Here's how the part is built. I have some questions about the finished solid (model axes, mm). A direction names the side the tool comes from. Give positions to 0.01 mm unless a question says otherwise; leave off trailing zeros. Write each loop counter-clockwise with the first axis right and the second up, starting at its lowest first coordinate (ties: lowest second). Pieces come first, ordered by that corner, then holes. Notation, with made-up numbers: M 40,-37 L 71,-37 A29 cw 71,-15 Z; hole C 34,33 d3. An arc over 180 degrees is marked long. Answer as CSV lines item,"result". Start each with the question number.
Q1. Suppose I cut it at C-C (z = 22). Write out the boundary of the cut face in (x, y).
Q2. Thinking about a two-plate mould opening in Y: for faces 1 (the cylindrical face through (5.009, -4.303, -13.206)), 2 (the cylindrical face through (6.26, -11.93, -10.25)), 3 (the cylindrical face through (6.26, 11.96, -10.3)), 4 (the cylindrical face through (5.009, 1.304, 15.728)), which applies, +Y half, -Y half, draft (parallel to the pull), parting line (faces both ways), or undercut?
Q3. Suppose I cut it at B-B (y = 0). Write out the boundary of the cut face in (x, z), then the cut area to 3 significant figures.
Q4. On a 3-axis mill with a long thin cutter (end or side, diameter ignored), from which of +Z, -Z, +X, -X, +Y, -Y can I reach the whole of each face in a straight line? I mean faces 5 (the cylindrical face through (6.261, -14.555, 6.101)), 6 (the flat face through (12.7, 0, 0)), 7 (the cylindrical face through (6.26, 8.18, 13.44)), 8 (the cylindrical face through (6.26, 10.3, 11.96)), 9 (the cylindrical face through (6.26, 11.93, 10.25)). Say none if no direction works.
Q5. If I drill on line 1 along Y through (x, z) = (9.25, -11.5); line 2 along Z through (x, y) = (3.25, 0.5); line 3 along Y through (x, z) = (1.5, 16.5), over which ranges is the centre line in solid material (lowest first)?
Q6. Suppose I cut it at A-A (z = 0). Write out the boundary of the cut face in (x, y).
Q7. For pin 1 (1.3 mm diameter, centred on x = 12, z = -22, fed in from +Y); pin 2 (3 mm diameter, centred on x = 1.5, z = -4.5, fed in from +Y); pin 3 (1.3 mm diameter, centred on x = 11, z = -20, fed in from -Y), each with a flat end and sliding along its axis, tell me the tip position at first contact or that it passes through.
```python
from build123d import *

# Parameters (mm, degrees)
BASPROSKE_W         = 12.7
BASPROSKE_H         = 17.4625
TOOTHCUT_DEPTH      = 28.769908399
TEETHCUTS_COUNT     = 20
TEETHCUTS_ANGLE     = 342
BORSKE_R            = 2.38125
BORE_DEPTH          = 50.8000508
SKETCH1_W           = 61.991981732
SKETCH1_H           = 12.955644482
BOSS_EXTRUDE1_DEPTH = 2.54


with BuildPart() as part:
    # BasProSke → Base-Revolve (revolve)
    with BuildSketch(Plane(origin=(0, 0, 0), x_dir=(1, 0, 0), z_dir=(0, 1, 0)), mode=Mode.PRIVATE) as base_revolve_sk:
        with Locations((6.35, 8.73125)):
            Rectangle(BASPROSKE_W, BASPROSKE_H)
    revolve(base_revolve_sk.sketch.rotate(Axis((-10, 0, 0), (1, 0, 0)), 180), axis=Axis((-10, 0, 0), (1, 0, 0)))

    # TooCutSke → ToothCut (cut, through all)
    with BuildSketch(Plane(origin=(0, 0, 0), x_dir=(0, 0, -1), z_dir=(1, 0, 0))):
        with BuildLine():
            ThreePointArc((0.788800759, 13.866938223), (0, 13.889355), (-0.788800759, 13.866938223))
            ThreePointArc((-0.788800759, 13.866938223), (-1.299448137, 15.717380814), (-2.339725589, 17.330675999))
            ThreePointArc((-2.339725589, 17.330675999), (0, 17.4879), (2.339725589, 17.330675999))
            ThreePointArc((2.339725589, 17.330675999), (1.299448137, 15.717380814), (0.788800759, 13.866938223))
        make_face()
    toothcut = extrude(amount=TOOTHCUT_DEPTH, mode=Mode.SUBTRACT)

    # TeethCuts: ToothCut ×20 about axis
    teethcuts_axis = Axis((-10, 0, 0), (1, 0, 0))
    for i in range(1, TEETHCUTS_COUNT):
        add(toothcut.rotate(teethcuts_axis, i * TEETHCUTS_ANGLE / (TEETHCUTS_COUNT - 1)), mode=Mode.SUBTRACT)

    # BorSke → Bore (cut, symmetric)
    with BuildSketch(Plane(origin=(0, 0, 0), x_dir=(0, 0, -1), z_dir=(1, 0, 0))):
        with Locations(Location((0, 0, 0), (0, 0, 180))):
            Circle(BORSKE_R)
    extrude(amount=BORE_DEPTH, both=True, mode=Mode.SUBTRACT)

    # Sketch1 → Boss-Extrude1 (add)
    with BuildSketch(Plane(origin=(12.7, 0, 0), x_dir=(0, 0, -1), z_dir=(1, 0, 0))):
        Rectangle(SKETCH1_W, SKETCH1_H)
    extrude(amount=-BOSS_EXTRUDE1_DEPTH)


solid = part.part
```
Resolved:
1,outline,"M 10.16,-6.48 L 12.7,-6.48 L 12.7,6.48 L 10.16,6.48 Z"
2,face 1,"undercut"
2,face 2,"-Y half"
2,face 3,"+Y half"
2,face 4,"undercut"
3,outline,"M 0,-13.89 L 10.16,-13.89 L 10.16,-31 L 12.7,-31 L 12.7,31 L 10.16,31 L 10.16,13.89 L 0,13.89 L 0,2.38 L 10.16,2.38 L 10.16,-2.38 L 0,-2.38 Z"
3,area,"391 mm^2"
4,face 5,"+X, -X, -Y"
4,face 6,"+Z, -Z, +X, +Y, -Y"
4,face 7,"+X, -X"
4,face 8,"+Z, +X, -X"
4,face 9,"+X, -X, +Y"
5,line 1,"-12.49 to -9.61, -7.79 to 7.79, 9.61 to 12.49"
5,line 2,"-13.88 to -2.33, 2.33 to 13.88"
5,line 3,"-3.39 to -1.72, 1.72 to 3.39"
6,outline,"M 0,-13.89 L 12.7,-13.89 L 12.7,13.89 L 0,13.89 L 0,2.38 L 10.16,2.38 L 10.16,-2.38 L 0,-2.38 Z"
7,pin 1,"y = 6.48"
7,pin 2,"y = 17.2"
7,pin 3,"y = -6.48"
